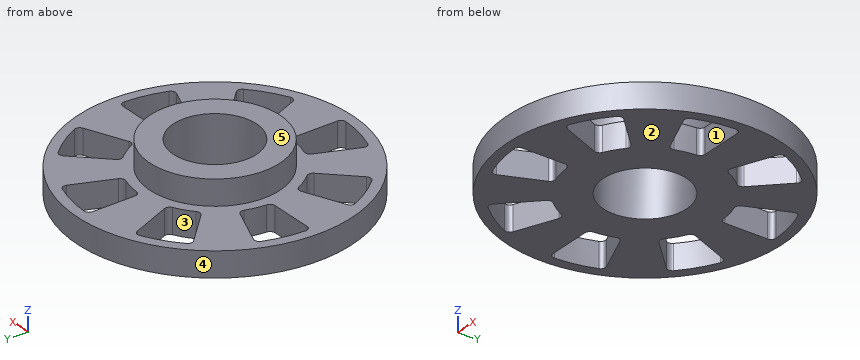
from build123d import *

# Parameters (mm, degrees)
SKETCH1_R                = 13.75
SKETCH1_R_2              = 4.15
BOSS_EXTRUDE1_DEPTH      = 2.5
SKETCH2_R                = 6.5
SKETCH2_R_2              = 4.15
BOSS_EXTRUDE2_DEPTH      = 2.5
CUT_EXTRUDE1_DEPTH       = 21.077973005
FILLET1_R                = 0.5
CIRPATTERN1_COUNT        = 8
FILLET1_OF_CIRPATTERN1_R = 0.5


with BuildPart() as part:
    # Sketch1 → Boss-Extrude1 (new body)
    with BuildSketch(Plane.XY):
        Circle(SKETCH1_R)
        Circle(SKETCH1_R_2, mode=Mode.SUBTRACT)
    extrude(amount=BOSS_EXTRUDE1_DEPTH)

    # Sketch2 → Boss-Extrude2 (add)
    with BuildSketch(Plane.XY.offset(2.5)):
        Circle(SKETCH2_R)
        Circle(SKETCH2_R_2, mode=Mode.SUBTRACT)
    extrude(amount=BOSS_EXTRUDE2_DEPTH)

    # Sketch5 → Cut-Extrude1 (cut, through all)
    with BuildSketch(Plane.XY):
        with BuildLine():
            Line((0, 12.75), (0, 7.5))
            ThreePointArc((0, 7.5), (1.463177415, 7.355889603), (2.870125743, 6.929096494))
            Line((2.870125743, 6.929096494), (4.879213763, 11.77946404))
            ThreePointArc((4.879213763, 11.77946404), (2.487401606, 12.505012325), (0, 12.75))
        make_face()
    cut_extrude1 = extrude(amount=CUT_EXTRUDE1_DEPTH, mode=Mode.SUBTRACT)

    # Fillet1
    fillet1_edges = [part.edges().sort_by_distance(p)[0] for p in [
        (0, 7.5, 1.25),
        (2.870125743, 6.929096494, 1.25),
        (4.879213763, 11.77946404, 1.25),
        (0, 12.75, 1.25),
    ]]
    fillet(fillet1_edges, radius=FILLET1_R)

    # CirPattern1: Cut-Extrude1 ×8 about axis
    cirpattern1_axis = Axis((0, 0, 0), (0, 0, 1))
    for i in range(1, CIRPATTERN1_COUNT):
        add(cut_extrude1.rotate(cirpattern1_axis, i * 360 / CIRPATTERN1_COUNT), mode=Mode.SUBTRACT)

    # Fillet1 of CirPattern1
    fillet1_of_cirpattern1_edges = [part.edges().sort_by_distance(p)[0] for p in [
        (-5.303300859, 5.303300859, 1.25),
        (-2.870125743, 6.929096494, 1.25),
        (-4.879213763, 11.77946404, 1.25),
        (-9.01561146, 9.01561146, 1.25),
        (-7.5, 0, 1.25),
        (-6.929096494, 2.870125743, 1.25),
        (-11.77946404, 4.879213763, 1.25),
        (-12.75, 0, 1.25),
        (-5.303300859, -5.303300859, 1.25),
        (-6.929096494, -2.870125743, 1.25),
        (-11.77946404, -4.879213763, 1.25),
        (-9.01561146, -9.01561146, 1.25),
        (0, -7.5, 1.25),
        (-2.870125743, -6.929096494, 1.25),
        (-4.879213763, -11.77946404, 1.25),
        (0, -12.75, 1.25),
        (5.303300859, -5.303300859, 1.25),
        (2.870125743, -6.929096494, 1.25),
        (4.879213763, -11.77946404, 1.25),
        (9.01561146, -9.01561146, 1.25),
        (7.5, 0, 1.25),
        (6.929096494, -2.870125743, 1.25),
        (11.77946404, -4.879213763, 1.25),
        (12.75, 0, 1.25),
        (5.303300859, 5.303300859, 1.25),
        (6.929096494, 2.870125743, 1.25),
        (11.77946404, 4.879213763, 1.25),
        (9.01561146, 9.01561146, 1.25),
    ]]
    fillet(fillet1_of_cirpattern1_edges, radius=FILLET1_OF_CIRPATTERN1_R)


solid = part.part
Model file for the job. Use its own axes, mm. Face numbers are marked on the shaded views. A direction names the side the tool comes from. Give positions to 0.01 mm unless a question says otherwise; leave off trailing zeros. Loops run counter-clockwise (first coordinate to the right, second up) from the corner with the lowest first, then second, coordinate; pieces in that order, holes last. Notation, with made-up numbers: (33, 57.5) -> (45, 57.5) arc R25 ccw to (45, 93.5) -> close; hole circle Ø7 at (79.5, 88.5). An arc over 180 degrees is marked (long way). Use a Markdown table: item, result. Add a question column.
(1) Mould opens along X. For the marked faces 3, 4 and 5 say: +X half, -X half, draft (parallel to the pull), parting line (faces both ways), or undercut.
(2) Drop flat-ended pins along their axis: pin 1 Ø3 at (y, z) = (-9, 1) entering from -X; pin 2 Ø3 at (x, z) = (10, 0.5) entering from -Y; pin 3 Ø1.2 at (y, z) = (10.5, 1) entering from +X. Give the stop position or say it passes through.
(3) Tool access for the marked faces 1 and 2: list every direction of +Z, -Z, +X, -X, +Y, -Y with a clear straight run to the whole face (end or side of a thin tool).
(4) Slice it at A-A on y = 10. List the corners of the cut face in (x, z), and give its area (3 significant figures).
(5) Slice it at C-C on z = 4.05. List the corners of the cut face in (x, y), and give its area (3 significant figures).
(6) Wall check: line 1 along Y through (x, z) = (0, 3.4); line 2 along X through (y, z) = (-1.75, 1.6); line 3 along Y through (x, z) = (-1, 2.45). Give the ranges that are in metal, low to high.
(7) Slice it at B-B on z = 1.3. Give the number of separate pieces and of enclosed holes in the cut face, and give its area (3 significant figures).
(8) Slice it at D-D on y = 6. List the corners of the cut face in (x, z).
Filled sheet:
| question | item | result |
|---|---|---|
| 1 | face 3 | undercut |
| 1 | face 4 | parting line |
| 1 | face 5 | draft |
| 2 | pin 1 | x = -11.52 |
| 2 | pin 2 | y = -10.81 |
| 2 | pin 3 | x = 9.54 |
| 3 | face 1 | +Z, -Z |
| 3 | face 2 | -Z, +X, -X, +Y, -Y |
| 4 | outline | (-9.44, 0) -> (-7.91, 0) -> (-7.91, 2.5) -> (-9.44, 2.5) -> close; (-4.14, 0) -> (0, 0) -> (0, 2.5) -> (-4.14, 2.5) -> close; (4.14, 0) -> (9.44, 0) -> (9.44, 2.5) -> (4.14, 2.5) -> close |
| 4 | area | 27.4 mm2 |
| 5 | outline | circle Ø13 at (0, 0); hole circle Ø8.3 at (0, 0) |
| 5 | area | 78.6 mm2 |
| 6 | line 1 | -6.5 to -4.15, 4.15 to 6.5 |
| 6 | line 2 | -13.64 to -3.76, 3.76 to 7.29, 12.63 to 13.64 |
| 6 | line 3 | -13.71 to -12.71, -7.43 to -4.03, 4.03 to 13.71 |
| 7 | separate pieces | 1 |
| 7 | enclosed holes | 9 |
| 7 | area | 375 mm2 |
| 8 | outline | (-12.37, 0) -> (-6, 0) -> (-6, 2.5) -> (-12.37, 2.5) -> close; (-4.5, 0) -> (6, 0) -> (6, 2.5) -> (2.5, 2.5) -> (2.5, 5) -> (-2.5, 5) -> (-2.5, 2.5) -> (-4.5, 2.5) -> close; (11.25, 0) -> (12.37, 0) -> (12.37, 2.5) -> (11.25, 2.5) -> close |
